Drawing for the job (mm, zero at the part's lowest x, y, z). A direction names the side the tool comes from. Coordinates: 2 decimals unless noted, no trailing zeros. Write each loop counter-clockwise with the first axis right and the second up, starting at its lowest first coordinate (ties: lowest second). Pieces come first, ordered by that corner, then holes. Notation, with made-up numbers: M 21.25,-18.75 L 80.25,-18.75 A28 ccw 80.25,12.25 Z; hole C 23.5,-22.75 d6. An arc over 180 degrees is marked long. Use a Markdown table: item, result. Add a question column.
Q1. Slice it at B-B on x = 30. Write the cut outline in (y, z), then the cut area to 4 significant figures.
Q2. Slice it at A-A on y = 42.5. Write the cut outline in (x, z), then the cut area to 3 significant figures.
Q3. Mould opens along Y. For the marked faces 1, 2, 3 and 4 say: released by +Y, released by -Y, zero draft, split by the parting line, or undercut.
Q4. Slice it at C-C on z = 1.4. Write the cut outline in (x, y).
Q5. Wall check: L1, parallel to X at y = 19.5, z = 1.1; L2, parallel to Y at x = 17.3, z = 2.95; L3, parallel to Y at x = 30, z = 2.05. Give the ranges that are in metal, low to high. Write a range as from..to.
Q6. Tool access for the marked faces 5, 6 and 7: list every direction of +Z, -Z, +X, -X, +Y, -Y with a clear straight run to the whole face (end or side of a thin tool).
Q7. Pin check, flat tips, straight feed: pin 1 Ø1.5 at (x, z) = (9.5, 3) entering from +Y; pin 2 Ø1.5 at (y, z) = (43, 3) entering from +X; pin 3 Ø1.5 at (x, z) = (20.5, 3.5) entering from +Y. Stop position of each tip, or through.
Q8. Slice it at D-D on y = 20. Write the cut outline in (x, z).
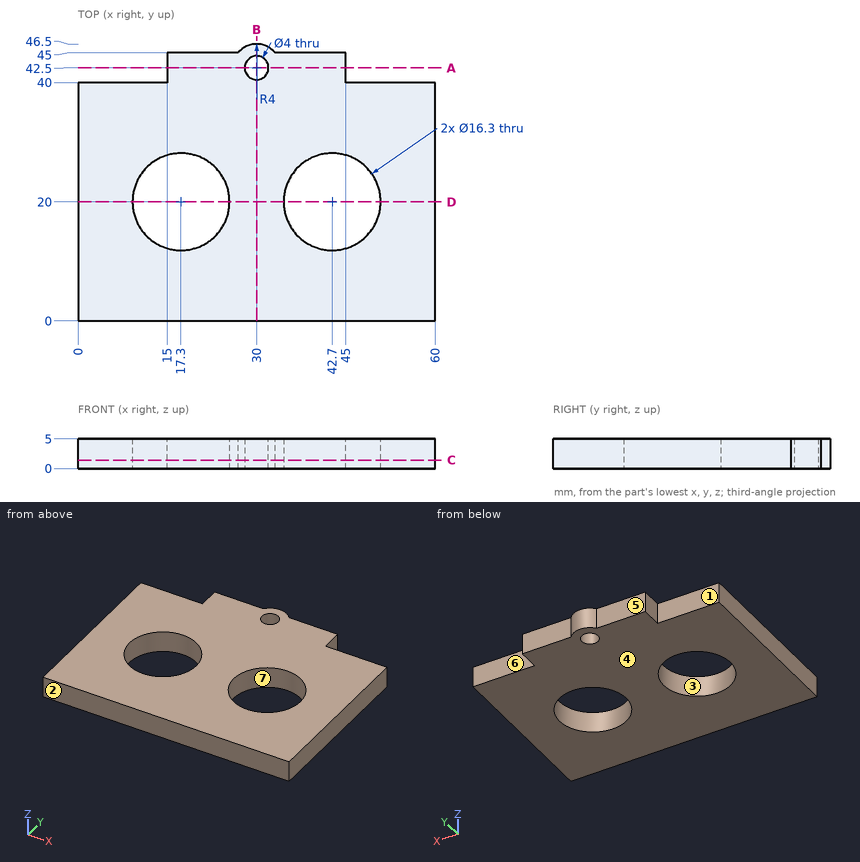
Recorded:
| question | item | result |
|---|---|---|
| 1 | outline | M 0,0 L 40.5,0 L 40.5,5 L 0,5 Z; M 44.5,0 L 46.5,0 L 46.5,5 L 44.5,5 Z |
| 1 | area | 212.5 mm² |
| 2 | outline | M 15,0 L 28,0 L 28,5 L 15,5 Z; M 32,0 L 45,0 L 45,5 L 32,5 Z |
| 2 | area | 130 mm² |
| 3 | face 1 | released by +Y |
| 3 | face 2 | released by -Y |
| 3 | face 3 | undercut |
| 3 | face 4 | zero draft |
| 4 | outline | M 0,0 L 60,0 L 60,40 L 45,40 L 45,45 L 33.12,45 A4 ccw 26.88,45 L 15,45 L 15,40 L 0,40 Z; hole C 17.3,20 d16.3; hole C 30,42.5 d4; hole C 42.7,20 d16.3 |
| 5 | L1 | 0..9.17, 25.43..34.57, 50.83..60 |
| 5 | L2 | 0..11.85, 28.15..45 |
| 5 | L3 | 0..40.5, 44.5..46.5 |
| 6 | face 5 | +Z, -Z, -X, +Y |
| 6 | face 6 | +Z, -Z, +X, +Y |
| 6 | face 7 | +Z, -Z |
| 7 | pin 1 | y = 40 |
| 7 | pin 2 | x = 45 |
| 7 | pin 3 | y = 45 |
| 8 | outline | M 0,0 L 9.15,0 L 9.15,5 L 0,5 Z; M 25.45,0 L 34.55,0 L 34.55,5 L 25.45,5 Z; M 50.85,0 L 60,0 L 60,5 L 50.85,5 Z |
